```python
from build123d import *

# Parameters (mm, degrees)
BOSS_EXTRUDE1_DEPTH = 8
SKETCH2_R           = 4
CUT_EXTRUDE1_DEPTH  = 44.462627624
BOSS_EXTRUDE2_DEPTH = 6
SKETCH5_R           = 12
BOSS_EXTRUDE3_DEPTH = 30
SKETCH8_R           = 6
CUT_EXTRUDE2_DEPTH  = 63.801273872
SKETCH9_W           = 30
SKETCH9_H           = 2
CUT_EXTRUDE3_DEPTH  = 63.801273872


with BuildPart() as part:
    # Sketch1 → Boss-Extrude1 (new body)
    with BuildSketch(Plane.XY):
        with BuildLine():
            Line((-33, -15), (40, -15))
            Line((40, -15), (40, 15))
            Line((40, 15), (-33, 15))
            ThreePointArc((-33, 15), (-37.949747468, 12.949747468), (-40, 8))
            Line((-40, 8), (-40, -8))
            ThreePointArc((-40, -8), (-37.949747468, -12.949747468), (-33, -15))
        make_face()
    extrude(amount=BOSS_EXTRUDE1_DEPTH)

    # Sketch2 → Cut-Extrude1 (cut, through all)
    with BuildSketch(Plane.XY.offset(8)):
        with Locations((-33, 0)):
            Circle(SKETCH2_R)
    extrude(amount=-CUT_EXTRUDE1_DEPTH, mode=Mode.SUBTRACT)

    # Sketch3 → Boss-Extrude2 (add)
    with BuildSketch(Plane(origin=(0, 15, 0), x_dir=(1, 0, 0), z_dir=(0, 1, 0))):
        Polygon((-8.722846682, 0), (40, 0), (40, 8), (20.815154113, 26), (-8.722846682, 26), align=None)
        Polygon((-8.722846682, 26), (20.815154113, 26), (11.487895334, 34.751212233), align=None)
    boss_extrude2 = extrude(amount=-BOSS_EXTRUDE2_DEPTH)

    # Mirror1: Boss-Extrude2 across plane
    add(boss_extrude2.mirror(Plane.ZX))

    # Sketch5 → Boss-Extrude3 (add, through all)
    with BuildSketch(Plane(origin=(0, 15, 0), x_dir=(1, 0, 0), z_dir=(0, 1, 0))):
        with Locations(Location((3.277153318, 26, 0), (0, 0, 180))):
            Circle(SKETCH5_R)
    extrude(amount=-BOSS_EXTRUDE3_DEPTH)

    # Sketch8 → Cut-Extrude2 (cut, through all)
    with BuildSketch(Plane(origin=(0, 15, 0), x_dir=(1, 0, 0), z_dir=(0, 1, 0))):
        with Locations(Location((3.277153318, 26, 0), (0, 0, 180))):
            Circle(SKETCH8_R)
    extrude(amount=-CUT_EXTRUDE2_DEPTH, mode=Mode.SUBTRACT)

    # Sketch9 → Cut-Extrude3 (cut, through all)
    with BuildSketch(Plane(origin=(0, 15, 0), x_dir=(1, 0, 0), z_dir=(0, 1, 0))):
        with Locations((0, -7)):
            Rectangle(SKETCH9_W, SKETCH9_H)
    extrude(amount=-CUT_EXTRUDE3_DEPTH, mode=Mode.SUBTRACT)


solid = part.part
```
Part model, mm, in its own coordinate system. A direction names the side the tool comes from. Give positions to 0.01 mm unless a question says otherwise; leave off trailing zeros. Order: outer loops, then holes, each group sorted by start corner. A loop starts at its lowest first (then second) coordinate and runs counter-clockwise, first axis right, second up. Notation, with made-up numbers: M 84,-31.75 L 91,-31.75 A23 cw 91,-8.75 Z; hole C 43.25,79.25 d5. An arc over 180 degrees is marked long. Use a Markdown table: item, result. Add a question column.
(1) Saw through at C-C, the plane x = 4. Give the cut face in (y, z).
(2) Saw through at A-A, the plane y = 0. Give the cut face in (x, z).
(3) Saw through at D-D, the plane z = 1. Give the cut face in (x, y), and give its area (3 significant figures).
(4) Probe line 1 along Y through (x, z) = (-8.5, -4); line 2 along Z through (x, y) = (23.5, -1.25); line 3 along Z through (x, y) = (-9.5, -11.5). List the from-to ranges inside material, lowest first. Write a range as [from, to].
(5) 3-axis set-ups, long thin cutter, end or side, ignore diameter. For faces 1 (the face through (0, 0, 6)), 2 (the face through (-9, 0, 0)), 3 (the face through (-8.723, -12, -13)), 4 (the face through (40, 0, 2)), 5 (the face through (-2.26, 0.21, -36.646)): which of +Z, -Z, +X, -X, +Y, -Y reach the whole face in a straight line?
(6) Mould opens along X. For faces 6 (the face through (-37.9, 13, 3.9)), 7 (the face through (-36.2, -2.4, 4.1)), 8 (the face through (11, 15, -10)) say: +X half, -X half, draft (parallel to the pull), parting line (faces both ways), or undercut.
(7) Saw through at B-B, the plane y = -5. Give the cut face in (x, z), and give its area (3 significant figures).
(8) Drop flat-ended pins along their axis: P1, Ø12, axis at x = 2.5, y = 0, coming from the +Z side; P2, Ø6.5, axis at y = -13.5, z = -15.5, coming from the -X side; P3, Ø6, axis at y = 10, z = -18.5, coming from the +X side. Give the stop position or say it passes through.
Answer key:
| question | item | result |
|---|---|---|
| 1 | outline | M -15,-37.98 L 15,-37.98 L 15,-31.96 L -15,-31.96 Z; M -15,-20.04 L 15,-20.04 L 15,6 L -15,6 Z; hole M -9,-14.02 L 9,-14.02 L 9,0 L -9,0 Z |
| 2 | outline | M -40,0 L -37,0 L -37,8 L -40,8 Z; M -29,0 L 40,0 L 40,8 L 15,8 L 15,6 L -15,6 L -15,8 L -29,8 Z; C 3.28,-26 d24; hole C 3.28,-26 d12 |
| 3 | outline | M -40,-8 A7 ccw -33,-15 L 40,-15 L 40,15 L -33,15 A7 ccw -40,8 Z; hole C -33,0 d8 |
| 3 | area | 2,330 mm^2 |
| 4 | line 1 | [-15, -9], [9, 15] |
| 4 | line 2 | [0, 8] |
| 4 | line 3 | [0, 6] |
| 5 | face 1 | +Z, +Y, -Y |
| 5 | face 2 | -X |
| 5 | face 3 | -Z, -X, +Y, -Y |
| 5 | face 4 | +Z, -Z, +X, +Y, -Y |
| 5 | face 5 | none |
| 6 | face 6 | -X half |
| 6 | face 7 | undercut |
| 6 | face 8 | draft |
| 7 | outline | M -40,0 L 40,0 L 40,8 L 15,8 L 15,6 L -15,6 L -15,8 L -40,8 Z; C 3.28,-26 d24; hole C 3.28,-26 d12 |
| 7 | area | 919 mm^2 |
| 8 | P1 | z = 6 |
| 8 | P2 | x = -8.72 |
| 8 | P3 | x = 32.01 |
